Design review of the part shown in the three views and the two pictorial views. Dimensions are in mm from the part's minimum x, y and z. Round coordinates to 2 decimals unless told otherwise and drop trailing zeros. Loops run counter-clockwise (first coordinate to the right, second up) from the corner with the lowest first, then second, coordinate; pieces in that order, holes last. Notation, with made-up numbers: (80, 75.25) -> (108, 75.25) arc R28 ccw to (108, 109.25) -> close; hole circle Ø3 at (45.25, 65). An arc over 180 degrees is marked (long way). Use a Markdown table: item, result. Add a question column.
1) Wall thickness on probe 1 along Y at (x, z) = (290, 46); probe 2 along Y at (x, z) = (117, 165.5); probe 3 along X at (y, z) = (545, 195): over which ranges is each line inside the solid? List them lowest first.
2) Mouldability with a two-part tool opening along X and no side actions: class the marked faces 1, 2 and 3 as released by +X, released by -X, zero draft, split by the parting line, or undercut.
3) Consider section A-A on x = 290. Give the boundary of the cut face in (y, z).
4) Insertion check: pin 1 (3 mm diameter, centred on y = 199.5, z = 128.5, fed in from +X); pin 2 (3 mm diameter, centred on x = 336.5, z = 77.5, fed in from -Y); pin 3 (5 mm diameter, centred on x = 322, z = 143.5, fed in from +Y); pin 4 (18 mm diameter, centred on x = 109.23, y = 470.77, fed in from -Z). Each pin has a flat end and moves straight along its axis. Give the tip position at first contact, or say it passes through.
5) Consider section C-C on x = 172. Give the boundary of the cut face in (y, z) (1 decimal).
6) Consider section D-D on y = 129.5. Give the boundary of the cut face in (x, z).
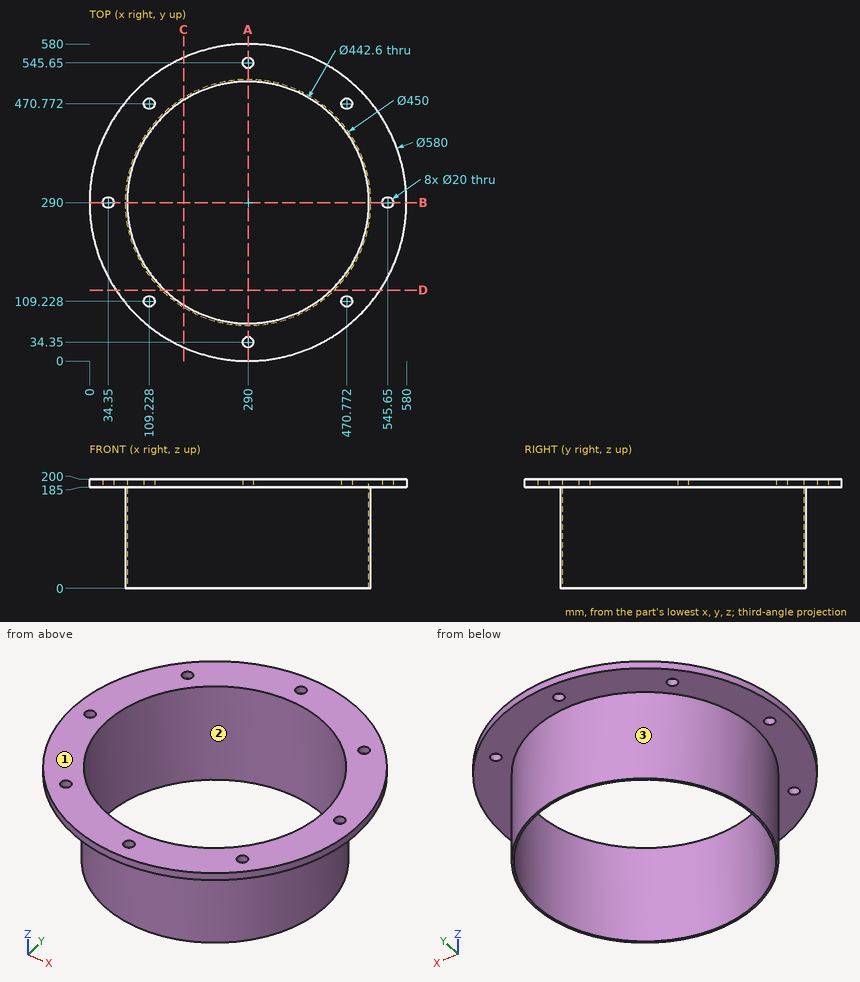
Result set:
| question | item | result |
|---|---|---|
| 1 | probe 1 | 65 to 68.7, 511.3 to 515 |
| 1 | probe 2 | 146.14 to 152, 428 to 433.86 |
| 1 | probe 3 | 151.89 to 280.02, 299.98 to 428.11 |
| 2 | face 1 | zero draft |
| 2 | face 2 | undercut |
| 2 | face 3 | split by the parting line |
| 3 | outline | (0, 185) -> (24.35, 185) -> (24.35, 200) -> (0, 200) -> close; (44.35, 185) -> (65, 185) -> (65, 0) -> (68.7, 0) -> (68.7, 200) -> (44.35, 200) -> close; (511.3, 0) -> (515, 0) -> (515, 185) -> (535.65, 185) -> (535.65, 200) -> (511.3, 200) -> close; (555.65, 185) -> (580, 185) -> (580, 200) -> (555.65, 200) -> close |
| 4 | pin 1 | x = 496.65 |
| 4 | pin 2 | y = 69.55 |
| 4 | pin 3 | y = 513.06 |
| 4 | pin 4 | through |
| 5 | outline | (25.1, 185) -> (98.4, 185) -> (98.4, 0) -> (102.8, 0) -> (102.8, 200) -> (25.1, 200) -> close; (477.2, 0) -> (481.6, 0) -> (481.6, 185) -> (554.9, 185) -> (554.9, 200) -> (477.2, 200) -> close |
| 6 | outline | (48.46, 185) -> (132.31, 185) -> (132.31, 0) -> (137.64, 0) -> (137.64, 200) -> (48.46, 200) -> close; (442.36, 0) -> (447.69, 0) -> (447.69, 185) -> (531.54, 185) -> (531.54, 200) -> (442.36, 200) -> close |
